```python
from build123d import *
from build123d.topology import SkipClean

# Parameters (mm, degrees)
SALIENTE_EXTRUIR1_DEPTH          = 7.5
TALADRO_DE_MARGEN_PARA_M61_D     = 6.4
TALADRO_DE_MARGEN_PARA_M61_DEPTH = 20
TALADRO_DE_MARGEN_PARA_M61_TIP   = 1.922753980888193
REDONDEO1_R                      = 2


with BuildPart() as part:
    # Croquis1 → Saliente-Extruir1 (new, symmetric)
    with SkipClean():  # the faces are left unmerged after this step: merging them gives an invalid solid
        with BuildSketch(Plane.XY):
            with BuildLine():
                Line((-14, 14), (-14, 0))
                ThreePointArc((-14, 1.71e-15), (-9.899494936611804, 9.899494936611527), (-3.9083e-13, 14))
                Line((-4.888e-14, 14), (-8.38e-14, 24))
                Line((-8.527e-14, 24.000000000000004), (-45, 24.000000000000004))
                Line((-45, 24.000000000000004), (-45, 14.000000000000005))
                Line((-45, 14.000000000000005), (-14, 14))
            make_face()
            with BuildLine():
                Line((-8.38e-14, 24), (-4.888e-14, 14))
                ThreePointArc((-3.9083e-13, 14), (9.899494936611529, 9.899494936611802), (14, 0))
                Line((14, 0), (14, 14))
                Line((14, 14), (45, 14.000000000000005))
                Line((45, 14.000000000000005), (45, 24.000000000000004))
                Line((45, 24.000000000000004), (-8.527e-14, 24.000000000000004))
            make_face()
            with BuildLine():
                ThreePointArc((-3.9083e-13, 14), (-9.899494936611804, 9.899494936611527), (-14, 1.71e-15))
                ThreePointArc((-14, 1.71e-15), (-9.89949493661153, -9.8994949366118), (3.829e-13, -14))
                Line((4.888e-14, -14), (2.793e-14, -8))
                ThreePointArc((-1.1516e-13, -8), (-8, -2.034e-14), (-1.5761e-13, 8))
                Line((-2.793e-14, 8), (-4.888e-14, 14))
            make_face()
            with BuildLine():
                ThreePointArc((14, 0), (9.899494936611529, 9.899494936611802), (-3.9083e-13, 14))
                Line((-4.888e-14, 14), (-2.793e-14, 8))
                ThreePointArc((-1.5761e-13, 8), (5.656854249492325, 5.656854249492436), (8, 0))
                ThreePointArc((8, -1.96e-15), (5.656854249492339, -5.656854249492421), (-1.1516e-13, -8))
                Line((2.793e-14, -8), (4.888e-14, -14))
                ThreePointArc((3.829e-13, -14), (9.899494936611795, -9.899494936611536), (14, -3.43e-15))
            make_face()
        extrude(amount=SALIENTE_EXTRUIR1_DEPTH, both=True)

    # Taladro de margen para M61
    with Locations(Plane(origin=(2.35e-15, 13.999999999999998, 0), x_dir=(-1, 2.6e-16, 0), z_dir=(-2.6e-16, -1, 0))):
        with Locations((22.5, 0), (-22.5, 0)):
            Hole(TALADRO_DE_MARGEN_PARA_M61_D / 2, depth=TALADRO_DE_MARGEN_PARA_M61_DEPTH)
            with Locations((0, 0, -(TALADRO_DE_MARGEN_PARA_M61_DEPTH + TALADRO_DE_MARGEN_PARA_M61_TIP / 2))):  # 118° drill point
                Cone(0, TALADRO_DE_MARGEN_PARA_M61_D / 2, TALADRO_DE_MARGEN_PARA_M61_TIP, mode=Mode.SUBTRACT)

    # Redondeo1
    redondeo1_edges = [part.edges().sort_by_distance(p)[0] for p in [
        (-14, 14, 0),
        (14, 14, 0),
    ]]
    fillet(redondeo1_edges, radius=REDONDEO1_R)


solid = part.part
```
Input: part model. Units: mm. Frame: model coordinates. A direction names the side the tool comes from. Coordinates: 2 decimals unless noted, no trailing zeros. Write each loop counter-clockwise with the first axis right and the second up, starting at its lowest first coordinate (ties: lowest second). Pieces come first, ordered by that corner, then holes. Notation, with made-up numbers: (67.5, 68) -> (100.5, 68) arc R8 cw to (100.5, 83) -> close; hole circle Ø7 at (-30.5, -5). An arc over 180 degrees is marked (long way). Write each question's results on one line, items separated by ' | '.
Item 1: Material intervals for probe 1 along X at (y, z) = (15.5, -2); probe 2 along Z at (x, y) = (-22.5, 17); probe 3 along Y at (x, z) = (-16, -5), sorted ascending.
Conclusion:
probe 1: x = -45 to -25, -20 to 20, 25 to 45 | probe 2: z = -7.5 to -3.2, 3.2 to 7.5 | probe 3: y = 14 to 24
Item 2: Section query B-B on z = 6. Return loops of the section in (x, y), plus the area to 3 significant figures.
Conclusion:
outline: (-45, 14) -> (-16, 14) arc R2 cw to (-14, 12) -> (-14, 0) arc R14 ccw to (14, 0) -> (14, 12) arc R2 cw to (16, 14) -> (45, 14) -> (45, 24) -> (-45, 24) -> close; hole circle Ø16 at (0, 0) | area: 1,400 mm^2
Item 3: Pin query (flat end, axial travel): pin 1 Ø3.5 at (y, z) = (5, 1.5) entering from +X; pin 2 Ø4.5 at (x, z) = (35, 0.5) entering from -Y; pin 3 Ø4 at (x, z) = (-22.5, 0) entering from +Y; pin 4 Ø6 at (y, z) = (4, -4) entering from -X. Return the tip coordinate at first contact, or that it passes through.
Conclusion:
pin 1: stops at x = 14 | pin 2: stops at y = 14 | pin 3: passes through | pin 4: stops at x = -14
Item 4: Section query D-D on x = -4. Return loops of the section in (y, z), plus the area to 3 significant figures.
Conclusion:
outline: (-13.42, -7.5) -> (-6.93, -7.5) -> (-6.93, 7.5) -> (-13.42, 7.5) -> close; (6.93, -7.5) -> (24, -7.5) -> (24, 7.5) -> (6.93, 7.5) -> close | area: 353 mm^2
Item 5: Set-up query: faces 1 (the flat face through (30, 14, 0)), 2 (the cylindrical face through (-25.7, 19.1, -0.1)). Return all of +Z, -Z, +X, -X, +Y, -Y with unobstructed straight access to the full face (end or side cutting, diameter ignored); none if empty.
Conclusion:
face 1: +Z, -Z, +X, -Y | face 2: +Y, -Y
Item 6: Section query C-C on y = 20. Return loops of the section in (x, z), plus the area to 3 significant figures.
Conclusion:
outline: (-45, -7.5) -> (45, -7.5) -> (45, 7.5) -> (-45, 7.5) -> close; hole circle Ø6.4 at (-22.5, 0); hole circle Ø6.4 at (22.5, 0) | area: 1,290 mm^2
Item 7: Section query A-A on x = 22.5. Return loops of the section in (y, z), plus the area to 3 significant figures.
Conclusion:
outline: (14, -7.5) -> (24, -7.5) -> (24, -3.2) -> (14, -3.2) -> close; (14, 3.2) -> (24, 3.2) -> (24, 7.5) -> (14, 7.5) -> close | area: 86.0 mm^2
Item 8: Mould query, pull axis Z, two halves, no side actions, for faces 3 (the flat face through (45, 19, 0)), 4 (the cylindrical face through (19.3, 19.1, -0.1)), 5 (the flat face through (-1, 14, -7.5)). Classes: +Z half, -Z half, draft (parallel to the pull), parting line (faces both ways), or undercut.
Conclusion:
face 3: draft | face 4: undercut | face 5: -Z half
